from build123d import *

# Parameters (mm, degrees)
F0_W     = 571.5
F0_H     = 50.8
F1_DEPTH = 19.05
F3_D     = 15.0114
F3_DEPTH = 14.224
F3_TIP   = 4.5098795482
F5_D     = 8.001
F5_DEPTH = 25.4
F5_TIP   = 2.4037429064


with BuildPart() as f1:
    # F0 (on Front) → F1 (new body)
    with BuildSketch(Plane.XZ):
        Rectangle(F0_W, F0_H)
    extrude(amount=F1_DEPTH)

    # F3
    with Locations(Plane(origin=(0, 0, 0), x_dir=(-1, 0, 0), z_dir=(0, 1, 0))):
        with Locations((234.95, 1.524), (0, 1.524), (-234.95, 1.524)):
            Hole(F3_D / 2, depth=F3_DEPTH)
            with Locations((0, 0, -(F3_DEPTH + F3_TIP / 2))):  # 118° drill point
                Cone(0, F3_D / 2, F3_TIP, mode=Mode.SUBTRACT)

    # F5
    with Locations(Plane.XY.offset(25.4)):
        with Locations((-234.95, -9.525), (0, -9.525), (234.95, -9.525)):
            Hole(F5_D / 2, depth=F5_DEPTH)
            with Locations((0, 0, -(F5_DEPTH + F5_TIP / 2))):  # 118° drill point
                Cone(0, F5_D / 2, F5_TIP, mode=Mode.SUBTRACT)


solid = f1.part
Can you work these out from the model? Positions are in its coordinate system, mm. A direction names the side the tool comes from. Coordinates: 2 decimals unless noted, no trailing zeros. Write item = value, one per line.
(1) For pin 1 (7 mm diameter, centred on x = -234.95, y = -9.525, fed in from +Z); pin 2 (9 mm diameter, centred on x = 0, z = 1.524, fed in from +Y); pin 3 (12 mm diameter, centred on x = 234.95, z = 1.524, fed in from +Y), each with a flat end and sliding along its axis, tell me the tip position at first contact or that it passes through.
Verdict:
pin_1 = -5.12
pin_2 = -16.03
pin_3 = -15.13
(2) If I drill on probe 1 along Z at (x, y) = (-234.95, -6.25); probe 2 along X at (y, z) = (-12.5, 6.5); probe 3 along Y at (x, z) = (234, 21), over which ranges is the centre line in solid material (lowest first)?
Verdict:
probe_1 = -25.4 to -5.98
probe_2 = -285.75 to -240.57, -229.33 to -5.62, 5.62 to 229.33, 240.57 to 285.75
probe_3 = -19.05 to -13.41, -5.64 to 0
(3) On a 3-axis mill with a long thin cutter (end or side, diameter ignored), from which of +Z, -Z, +X, -X, +Y, -Y can I reach the whole of each face in a straight line? I mean faces 1 (the face through (-236.6, -7.2, -5.8)), 2 (the face through (-4, -12, 25.4)). Say none if no direction works.
Verdict:
face_1 = +Y
face_2 = +Z, +X, -X, +Y, -Y
(4) Thinking about a two-plate mould opening in X: for faces 3 (the face through (-4, -19.05, 0)), 4 (the face through (-1.24, -17.95, 1.92)), 5 (the face through (-285.75, -9, 0)), which applies, +X half, -X half, draft (parallel to the pull), parting line (faces both ways), or undercut?
Verdict:
face_3 = draft
face_4 = undercut
face_5 = -X half
